The model under review builds one solid part; all positions refer to its coordinate system, in mm. A direction names the side the tool comes from. Give positions to 0.01 mm unless a question says otherwise; leave off trailing zeros. Loops run counter-clockwise (first coordinate to the right, second up) from the corner with the lowest first, then second, coordinate; pieces in that order, holes last. Notation, with made-up numbers: (-14.5, 52.5) - (11.5, 52.5) arc R32 ccw to (11.5, 87.5) - close; hole circle Ø2 at (6.25, -22.75). An arc over 180 degrees is marked (long way). Return JSON: item names as keys, results as strings. Group by question number.
from build123d import *

# Parameters (mm, degrees)
F1_DEPTH = 203.2
F2_R     = 3.175
F3_DEPTH = 101.6
F4_R     = 3.175
F5_DEPTH = 25.4


with BuildPart() as f1:
    # F0 (on Front) → F1 (new body)
    with BuildSketch(Plane.XZ):
        Polygon((53.975, 44.519556), (0, 44.519556), (0, -35.871444), (34.925, -35.871444), (34.925, -32.696444), (3.175, -32.696444), (3.175, 41.344556), (53.975, 41.344556), align=None)
    extrude(amount=F1_DEPTH)

    # F2 (on face) → F3 (cut)
    with BuildSketch(Plane.XY.offset(44.519556)):
        with Locations((41.275, -190.5)):
            Circle(F2_R)
        with Locations((41.275, -165.1)):
            Circle(F2_R)
        with Locations((41.275, -139.7)):
            Circle(F2_R)
        with Locations((41.275, -114.3)):
            Circle(F2_R)
        with Locations((41.275, -88.9)):
            Circle(F2_R)
        with Locations((41.275, -63.5)):
            Circle(F2_R)
        with Locations((41.275, -38.1)):
            Circle(F2_R)
        with Locations((41.275, -12.7)):
            Circle(F2_R)
        with Locations((15.875, -190.5)):
            Circle(F2_R)
        with Locations((15.875, -165.1)):
            Circle(F2_R)
        with Locations((15.875, -139.7)):
            Circle(F2_R)
        with Locations((15.875, -114.3)):
            Circle(F2_R)
        with Locations((15.875, -88.9)):
            Circle(F2_R)
        with Locations((15.875, -63.5)):
            Circle(F2_R)
        with Locations((15.875, -38.1)):
            Circle(F2_R)
        with Locations((15.875, -12.7)):
            Circle(F2_R)
    extrude(amount=-F3_DEPTH, mode=Mode.SUBTRACT)

    # F4 (on face) → F5 (cut)
    with BuildSketch(Plane.XY.offset(44.519556)):
        with BuildLine():
            Line((15.875, -184.15), (53.975, -184.15))
            Line((53.975, -184.15), (53.975, -133.35))
            Line((53.975, -133.35), (15.875, -133.35))
            Line((15.875, -133.35), (15.875, -136.525))
            ThreePointArc((15.875, -136.525), (18.120064, -137.454936), (19.05, -139.7))
            ThreePointArc((19.05, -139.7), (18.120064, -141.945064), (15.875, -142.875))
            Line((15.875, -142.875), (15.875, -161.925))
            ThreePointArc((15.875, -161.925), (18.120064, -162.854936), (19.05, -165.1))
            ThreePointArc((19.05, -165.1), (18.120064, -167.345064), (15.875, -168.275))
            Line((15.875, -168.275), (15.875, -184.15))
        make_face()
        with Locations((41.275, -165.1)):
            Circle(F4_R, mode=Mode.SUBTRACT)
        with Locations((41.275, -139.7)):
            Circle(F4_R, mode=Mode.SUBTRACT)
    extrude(amount=-F5_DEPTH, mode=Mode.SUBTRACT)


solid = f1.part
Item 1: For L1, parallel to X at y = -114, z = 43 (3 decimals); L2, parallel to Z at x = 20, y = -125; L3, parallel to X at y = -170, z = -11.5 (3 decimals), list the stretches that pass through material, from the lowest coordinate up. Write a range as from..to.
Item 2: For P1, Ø1, axis at y = -92, z = -34, coming from the +X side (3 decimals); P2, Ø5, axis at y = -69.5, z = 6.5, coming from the +X side (3 decimals); P3, Ø2.5, axis at y = -135, z = 42.5, coming from the +X side (3 decimals), all flat-tipped, find the tip position at first contact; note any pin that passes through.
Item 3: Mouldability with a two-part tool opening along Y and no side actions: class faces 1 (the face through (18.808, -13.916, -34.262)), 2 (the face through (17.58, -60.82, 42.95)), 3 (the face through (28, -78, 41.345)) as +Y half, -Y half, draft (parallel to the pull), parting line (faces both ways), or undercut.
Item 4: Take a section at D-D (y = -106). State the section outline as (x, z) points (3 decimals), then the cut area to 3 significant figures.
Item 5: Take a section at A-A (y = -38.1). State the section outline as (x, z) points (3 decimals), then the cut area to 3 significant figures.
Item 6: Take a section at B-B (x = 10.5). State the section outline as (y, z) points.
Item 7: Take a section at C-C (y = -139.7). State the section outline as (x, z) points (3 decimals).
Item 8: Tool access review of faces 4 (the face through (15.462, -187.352, 42.954)), 5 (the face through (3.175, -100, 4)): name each direction out of +Z, -Z, +X, -X, +Y, -Y from which nothing blocks a thin tool from reaching the whole face with its end or side.
Check sheet entries:
{
 "1": {"L1": "x = 0..12.714, 19.036..38.114, 44.436..53.975", "L2": "z = -35.87..-32.7, 41.34..44.52", "L3": "x = 0..3.175"},
 "2": {"P1": "stops at x = 34.925", "P2": "stops at x = 3.175", "P3": "stops at x = 15.875"},
 "3": {"face 1": "undercut", "face 2": "undercut", "face 3": "draft"},
 "4": {"outline": "(0, -35.871) - (34.925, -35.871) - (34.925, -32.696) - (3.175, -32.696) - (3.175, 41.345) - (53.975, 41.345) - (53.975, 44.52) - (0, 44.52) - close", "area": "517 mm^2"},
 "5": {"outline": "(0, -35.871) - (12.7, -35.871) - (12.7, -32.696) - (3.175, -32.696) - (3.175, 41.345) - (12.7, 41.345) - (12.7, 44.52) - (0, 44.52) - close; (19.05, -35.871) - (34.925, -35.871) - (34.925, -32.696) - (19.05, -32.696) - close; (19.05, 41.345) - (38.1, 41.345) - (38.1, 44.52) - (19.05, 44.52) - close; (44.45, 41.345) - (53.975, 41.345) - (53.975, 44.52) - (44.45, 44.52) - close", "area": "457 mm^2"},
 "6": {"outline": "(-203.2, -35.87) - (0, -35.87) - (0, -32.7) - (-203.2, -32.7) - close; (-203.2, 41.34) - (0, 41.34) - (0, 44.52) - (-203.2, 44.52) - close"},
 "7": {"outline": "(0, -35.871) - (12.7, -35.871) - (12.7, -32.696) - (3.175, -32.696) - (3.175, 41.345) - (12.7, 41.345) - (12.7, 44.52) - (0, 44.52) - close; (19.05, -35.871) - (34.925, -35.871) - (34.925, -32.696) - (19.05, -32.696) - close"},
 "8": {"face 4": "+Z, -Z", "face 5": "+X, +Y, -Y"}
}
